from build123d import *

# Parameters (mm, degrees)
F1_DEPTH = 50
F2_R     = 50
F3_R     = 30
F4_R     = 20
F5_R     = 5
F6_R     = 5


with BuildPart() as f1:
    # F0 (on Front) → F1 (new body)
    with BuildSketch(Plane.XZ):
        Polygon((-23.6634109169, 31.7528273398), (0, -41.8914239646), (35.305287689, -41.8914239646), (35.305287689, -33.2806184888), (8.2252407447, -33.2806184888), (8.2252407447, -15.5646987259), (34.3599072305, -15.5646987259), (34.3599072305, -6.3414066872), (4.1758916341, 4.428982269), (-23.6634109169, 44.6694269776), (-62.7042563281, 44.6694269776), (-62.7042563281, 41.6324101388), align=None)
    extrude(amount=F1_DEPTH)

    # F2
    f2_edges = [f1.edges().sort_by_distance(p)[0] for p in [
        (4.175892, -25, 4.428982),
    ]]
    fillet(f2_edges, radius=F2_R)

    # F3
    f3_edges = [f1.edges().sort_by_distance(p)[0] for p in [
        (-23.663411, -25, 31.752827),
    ]]
    fillet(f3_edges, radius=F3_R)

    # F4
    f4_edges = [f1.edges().sort_by_distance(p)[0] for p in [
        (0, -25, -41.891424),
    ]]
    fillet(f4_edges, radius=F4_R)

    # F5
    f5_edges = [f1.edges().sort_by_distance(p)[0] for p in [
        (35.305288, -25, -41.891424),
        (34.359907, -25, -6.341407),
        (2.798647, 0, -38.052587),
        (-4.460469, -25, -28.009743),
        (14.580701, -25, -41.891424),
        (2.798647, -50, -38.052587),
    ]]
    fillet(f5_edges, radius=F5_R)

    # F6
    f6_edges = [f1.edges().sort_by_distance(p)[0] for p in [
        (-14.322206, -50, 31.16714),
        (5.713271, 0, 6.433938),
    ]]
    fillet(f6_edges, radius=F6_R)


solid = f1.part
Verification items for the finished model (mm, model axes). A direction names the side the tool comes from. Coordinates: 2 decimals unless noted, no trailing zeros. Write each loop counter-clockwise with the first axis right and the second up, starting at its lowest first coordinate (ties: lowest second). Pieces come first, ordered by that corner, then holes. Notation, with made-up numbers: M 50.5,25 L 92.5,25 A28 ccw 92.5,52 Z; hole C 58.25,-7 d11. An arc over 180 degrees is marked long. Use CSV: the item, a comma, the result in double quotes.
Q1. Thickness scan on line 1 along Z through (x, y) = (27.5, -19); line 2 along Z through (x, y) = (24, -35); line 3 along X through (y, z) = (-8.5, 15.5). Record the ranges inside material, lowest first. Write a range as [from, to].
Computed values:
line 1,"[-41.89, -33.28], [-15.56, -3.89]"
line 2,"[-41.89, -33.28], [-15.56, -2.64]"
line 3,"[-18.44, -3.4]"
Q2. Set-up check for faces 4 (the flat face through (21, -25, -15.565)), 5 (the flat face through (0, 0, -5)), 6 (the flat face through (34.36, -25, -13)): record each of +Z, -Z, +X, -X, +Y, -Y from which the full face is reachable in a straight line by a thin tool's end or side.
Computed values:
face 4,"+X, +Y, -Y"
face 5,"+Z, -Z, +X, -X, +Y"
face 6,"+Z, +X, +Y, -Y"
Q3. Mould release check, pull along Z, two halves, no side actions. Record for faces 1 (the flat face through (8.225, -25, -25)), 2 (the cylindrical face through (24.626, -48.496, -4.382)), 3 (the cylindrical face through (25.09, -1.43, -40.39)): pulls with the +Z half, pulls with the -Z half, needs draft (parallel to the pull), parting line crosses it, or undercut.
Computed values:
face 1,"undercut"
face 2,"pulls with the +Z half"
face 3,"pulls with the -Z half"
Q4. Section check A-A, the plane y = -10. Enter the section's corners in (x, z).
Computed values:
outline,"M -62.7,41.63 L -39.78,35.83 A30 cw -18.58,15.93 L -4.46,-28.01 A20 ccw 14.58,-41.89 L 30.31,-41.89 A5 ccw 35.31,-36.89 L 35.31,-33.28 L 8.23,-33.28 L 8.23,-15.56 L 34.36,-15.56 L 34.36,-9.87 A5 ccw 31.04,-5.16 L 19.33,-0.98 A50 cw -4.98,17.66 L -23.66,44.67 L -62.7,44.67 Z"
Q5. Go/stop test with flat-tipped pins: P1, Ø6, axis at x = -43, z = 31.5, coming from the +Y side; P2, Ø13.5, axis at x = 22.5, y = -15.5, coming from the +Z side; P3, Ø3, axis at x = -41.5, z = 35.5, coming from the +Y side; P4, Ø1.5, axis at x = 12.5, y = -14.5, coming from the +Z side. Record where each tip stops, or that it passes through.
Computed values:
P1,"through"
P2,"z = 0.46"
P3,"y = -2.35"
P4,"z = 2.46"
